The listing builds one solid part. Answer for the finished solid, in the listing's coordinates (mm). A direction names the side the tool comes from. Coordinates: 2 decimals unless noted, no trailing zeros. Order: outer loops, then holes, each group sorted by start corner. A loop starts at its lowest first (then second) coordinate and runs counter-clockwise, first axis right, second up. Notation, with made-up numbers: (-10, 14) - (28, 14) arc R9 cw to (28, 25) - close; hole circle Ø6 at (-10.75, 71). An arc over 180 degrees is marked (long way). Use one line per item in the form item = value. Start each with the question number.
Item 1: Section D-D, the plane x = 15.25 is taken. Write down the section's boundary in (y, z), and give its area (3 significant figures).
Item 2: Section C-C, the plane z = 26 is taken. Write down the section's boundary in (x, y), and give its area (3 significant figures).
Item 3: Each of these flat-tipped pins is pushed along its axis until it touches: pin 1 Ø3 at (y, z) = (-23.5, 44.5) entering from +X; pin 2 Ø1.2 at (x, z) = (5.5, 1.5) entering from -Y; pin 3 Ø1 at (x, y) = (5, 8) entering from -Z; pin 4 Ø1.5 at (y, z) = (-7, 6) entering from +X. Where does it stop, or does it pass through?
Item 4: The mould has two halves that part along Z. Classify faces 4 (the cylindrical face through (23.43, -13.52, 45.4)), 5 (the flat face through (2, -36, 9.5)), 6 (the flat face through (2, -47, 5)), 7 (the cylindrical face through (2.028, 12.677, 34.351)): released by +Z, released by -Z, zero draft, split by the parting line, or undercut.
Item 5: Section A-A, the plane z = 34 is taken. Write down the section's boundary in (x, y), and give its area (3 significant figures).
Item 6: Consider line 1 along Y through (x, z) = (2.1, 34); line 2 along Y through (x, z) = (3.25, 7); line 3 along Y through (x, z) = (4.25, 36). Determine where each line is inside the solid, lowest interval first. Write a range as [from, to].
Item 7: A tool of negligible diameter and unlimited length cuts with its end or side. For faces 1 (the flat face through (8, -22, 2.5)), 2 (the flat face through (13, -22, 45)), 3 (the flat face through (4, 4, 23)), from which of +Z, -Z, +X, -X, +Y, -Y can it reach the whole face along a straight path? Write none if from no direction.
Item 8: Section B-B, the plane y = 10 is taken. Write down the section's boundary in (x, z), and give its area (3 significant figures).
Autodesk Fusion 360 part; units mm, degrees
sketch "Sketch1" plane through (0, 0, 0) normal (0, 0, 1) x (1, 0, 0)
  line L0 (4, 0) -> (4, 20)
  line L1 (4, 20) -> (0, 20)
  line L2 (0, 20) -> (0, 0)
  line L3 (0, 0) -> (4, 0)
  line L4 (4, 0) -> (4, -15)
  line L5 (4, -15) -> (0, -15)
  line L6 (0, -15) -> (0, 0)
  line L7 (0, -15) -> (3, -15)
  line L8 (3, -15) -> (3, -47)
  line L9 (3, -47) -> (0, -47)
  line L10 (0, -47) -> (0, -15)
  dimension "d1" = 20
  dimension "d2" = 4
  dimension "d3" = 15
  dimension "d4" = 32
  dimension "d5" = 3
extrude "Extrude1" add sketch "Sketch1" along normal blind 46
sketch "Sketch2" plane through (4, 0, 0) normal (1, 0, 0) x (0, 0, -1)
  line L0 (0, -15) -> (0, 20)
  line L1 (0, 20) -> (-46, 20)
  line L2 (-46, 20) -> (-46, -15)
  line L3 (-46, -15) -> (0, -15)
  line L4 (-46, 10) -> (0, 10) construction
  circle A0 centre (-34, 10) radius 2.7
  circle A1 centre (-7, 10) radius 2.7
  line L5 (-46, -12) -> (0, -12)
  line L6 (0, -47) -> (0, -15) construction
  line L7 (0, -15) -> (-46, -15) construction
  line L8 (-46, -15) -> (-46, -47) construction
  line L9 (-46, -47) -> (0, -47) construction
  line L10 (-23, 20) -> (-23, -47) construction
  line L11 (-36.5, -25) -> (-9.5, -25)
  line L12 (-9.5, -25) -> (-9.5, -47)
  line L13 (-9.5, -47) -> (-36.5, -47)
  line L14 (-36.5, -47) -> (-36.5, -25)
  dimension "d8" = 5.4
  dimension "d9" = 5.4
  dimension "d10" = 3
  dimension "d11" = 27
  dimension "d12" = 22
  dimension "d17" = 7
  dimension "d18" = 12
  dimension "d19" = 11.5
  dimension "d24" = 25
  dimension "d25" = 15
extrude "Extrude3" add sketch "Sketch2" along normal blind 20 contours L0 L2 L3 L5
extrude "Extrude2" cut sketch "Sketch2" against normal through all contours A0 | A1 | L11 L12 L13 L14
sketch "Sketch3" plane through (3, 0, 0) normal (1, 0, 0) x (0, 0, -1)
  line L0 (-9.5, -25) -> (-9.5, -47)
  line L1 (-9.5, -47) -> (0, -47)
  line L2 (0, -47) -> (0, -15)
  line L3 (0, -15) -> (-46, -15)
  line L4 (-46, -15) -> (-46, -47)
  line L5 (-46, -47) -> (-36.5, -47)
  line L6 (-36.5, -47) -> (-36.5, -25)
  line L7 (-36.5, -25) -> (-9.5, -25)
  line L8 (-46, -15) -> (-43.5, -15)
  line L9 (-43.5, -15) -> (-43.5, -30)
  line L10 (-43.5, -30) -> (-46, -30)
  line L11 (-46, -30) -> (-46, -15)
  line L12 (0, -15) -> (-2.5, -15)
  line L13 (-2.5, -15) -> (-2.5, -30)
  line L14 (-2.5, -30) -> (0, -30)
  line L15 (0, -30) -> (0, -15)
  dimension "d26" = 15
  dimension "d27" = 2.5
  dimension "d28" = 2.5
extrude "Extrude4" add sketch "Sketch3" along normal blind 10 contours L2 L3 L12 L13 L14 L15 | L3 L4 L8 L9 L10 L11
fillet "Fillet1" radius 2 4 edges at (2, 20, 46) (2, 20, 0) (24, -13.5, 0) (24, -13.5, 46)
fillet "Fillet2" radius 1 8 edges at (1.5, -25, 36.5) (1.5, -25, 9.5) (1.5, -47, 9.5) (1.5, -47, 0) (1.5, -47, 36.5) (1.5, -47, 46) (13, -30, 44.75) (13, -30, 1.25)
equation "d9 = d8"
equation "d28 = d27"
Response:
q1.outline = (-15, 0) - (-12, 0) - (-12, 46) - (-15, 46) - close
q1.area = 138 mm2
q2.outline = (0, -25) - (3, -25) - (3, -15) - (24, -15) - (24, -12) - (4, -12) - (4, 20) - (0, 20) - close
q2.area = 230 mm2
q3.pin_1 = 13
q3.pin_2 = -30
q3.pin_3 = through
q3.pin_4 = 4
q4.face_4 = released by +Z
q4.face_5 = undercut
q4.face_6 = zero draft
q4.face_7 = undercut
q5.outline = (0, -25) - (3, -25) - (3, -15) - (24, -15) - (24, -12) - (4, -12) - (4, 7.3) - (0, 7.3) - close; (0, 12.7) - (4, 12.7) - (4, 20) - (0, 20) - close
q5.area = 208 mm2
q6.line_1 = [-25, 7.3], [12.7, 20]
q6.line_2 = [-15, 7.3], [12.7, 20]
q6.line_3 = [-15, -12]
q7.face_1 = +X, -Y
q7.face_2 = +Z, -Z, +X, -Y
q7.face_3 = +Z, -Z, +X, +Y
q8.outline = (0, 0) - (4, 0) - (4, 4.3) - (0, 4.3) - close; (0, 9.7) - (4, 9.7) - (4, 31.3) - (0, 31.3) - close; (0, 36.7) - (4, 36.7) - (4, 46) - (0, 46) - close
q8.area = 141 mm2
